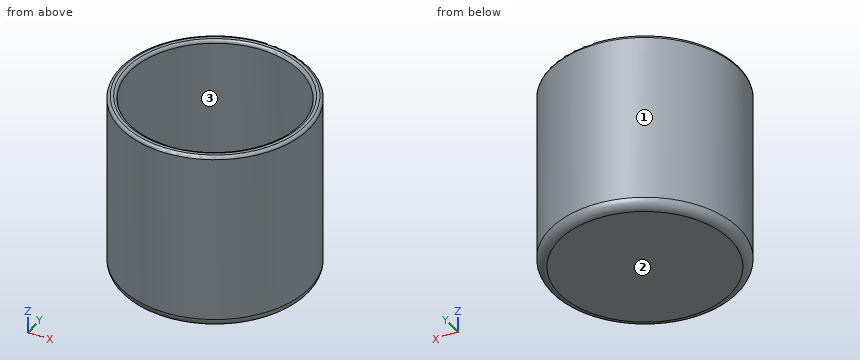
from build123d import *

# Parameters (mm, degrees)
F2_R = 1
F3_R = 1


with BuildPart() as f1:
    # F0 (on Front) → F1 (revolve)
    with BuildSketch(Plane.XZ):
        with BuildLine():
            Line((25.776508, -31.088909), (0, -31.088909))
            Line((0, -31.088909), (0, -34.088909))
            Line((0, -34.088909), (28.776508, -34.088909))
            ThreePointArc((28.776508, -34.088909), (30.897828, -33.210229), (31.776508, -31.088909))
            Line((31.776508, -31.088909), (31.776508, 26.721045))
            Line((31.776508, 26.721045), (28.776508, 26.721045))
            Line((28.776508, 26.721045), (28.776508, -28.088909))
            ThreePointArc((28.776508, -28.088909), (27.897828, -30.210229), (25.776508, -31.088909))
        make_face()
    revolve(axis=Axis((0, 0, -7.964928), (0, 0, -1)))

    # F2
    f2_edges = [f1.edges().sort_by_distance(p)[0] for p in [
        (-28.776508, 0, 26.721045),
    ]]
    fillet(f2_edges, radius=F2_R)

    # F3
    f3_edges = [f1.edges().sort_by_distance(p)[0] for p in [
        (-31.776508, 0, 26.721045),
    ]]
    fillet(f3_edges, radius=F3_R)


solid = f1.part
For this review, take the finished solid that the model builds, in its own axes (mm). Face numbers are marked on the shaded views. Give positions to 0.01 mm unless a question says otherwise; leave off trailing zeros. Order: outer loops, then holes, each group sorted by start corner. A loop starts at its lowest first (then second) coordinate and runs counter-clockwise, first axis right, second up. Notation, with made-up numbers: (21.25, -6.75) - (58.25, -6.75) arc R31 ccw to (58.25, 29.25) - close; hole circle Ø4 at (68, 70.25). An arc over 180 degrees is marked (long way). Answer as a JSON object with one key per item and string values. Group by question number.
Item 1: Take a section at C-C on z = -24.5. Give the boundary of the cut face in (x, y), and give its area (3 significant figures).
Item 2: Wall thickness on line 1 along Y through (x, z) = (0, 0.5); line 2 along Z through (x, y) = (-12.5, 24): over which ranges is each line inside the solid? List them lowest first.
Item 3: Clearance check with flat-ended pins moving along their axes: pin 1 Ø1.5 at (y, z) = (-8, -25) entering from +X; pin 2 Ø8 at (y, z) = (11, 5) entering from +X; pin 3 Ø1 at (y, z) = (22.5, -24) entering from -X. State where each tip first meets the part, or that it passes through.
Item 4: Draft analysis for pull direction X (two halves, no side actions). For the marked faces 1, 2 and 3, state which applies: pulls with the +X half, pulls with the -X half, needs draft (parallel to the pull), parting line crosses it, or undercut.
Item 5: Take a section at A-A on y = 0. Give the boundary of the cut face in (x, z).
Reported:
{
 "1": {"outline": "circle Ø63.55 at (0, 0); hole circle Ø57.55 at (0, 0)", "area": "571 mm^2"},
 "2": {"line 1": "-31.78 to -28.78, 28.78 to 31.78", "line 2": "-34.09 to -30.8"},
 "3": {"pin 1": "x = 30.94", "pin 2": "x = 31", "pin 3": "x = -22.93"},
 "4": {"face 1": "parting line crosses it", "face 2": "needs draft", "face 3": "undercut"},
 "5": {"outline": "(-31.78, -31.09) arc R3 ccw to (-28.78, -34.09) - (28.78, -34.09) arc R3 ccw to (31.78, -31.09) - (31.78, 25.72) arc R1 ccw to (30.78, 26.72) - (29.78, 26.72) arc R1 ccw to (28.78, 25.72) - (28.78, -28.09) arc R3 cw to (25.78, -31.09) - (-25.78, -31.09) arc R3 cw to (-28.78, -28.09) - (-28.78, 25.72) arc R1 ccw to (-29.78, 26.72) - (-30.78, 26.72) arc R1 ccw to (-31.78, 25.72) - close"}
}
